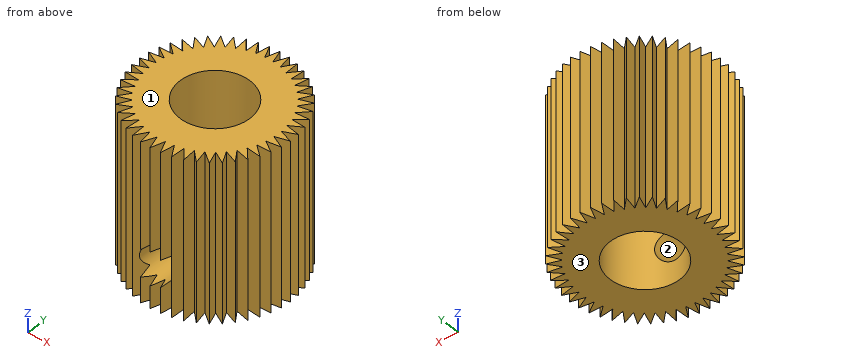
from build123d import *

# Parameters (mm, degrees)
EXTRUDE_1_DEPTH   = 11.4
OTHER_1_OUTLINE_R = 2.5
OTHER_1_DEPTH     = 11.4
SKETCH_9_R        = 1.2


# Read off the part's stored shape, not the designer's step: 孔1
with BuildPart() as part:
    # 草图6 → 凸台-拉伸1 (new body)
    with BuildSketch(Plane.XY):
        Polygon((5.393460046, -0.710062486), (4.490365155, -0.294314082), (5.44, 0), (4.490365155, 0.294314082), (5.393460046, 0.710062486), (4.413533762, 0.877906449), (5.254636495, 1.407975605), (4.261185583, 1.446477594), (5.025904657, 2.081797872), (4.035927337, 1.990299106), (4.711178197, 2.72), (3.741613255, 2.500066049), (4.315842171, 3.311662174), (3.383279134, 2.967056168), (3.84666089, 3.84666089), (2.967056168, 3.383279134), (3.311662174, 4.315842171), (2.500066049, 3.741613255), (2.72, 4.711178197), (1.990299106, 4.035927337), (2.081797872, 5.025904657), (1.446477594, 4.261185583), (1.407975605, 5.254636495), (0.877906449, 4.413533762), (0.710062486, 5.393460046), (0.294314082, 4.490365155), (0, 5.44), (-0.294314082, 4.490365155), (-0.710062486, 5.393460046), (-0.877906449, 4.413533762), (-1.407975605, 5.254636495), (-1.446477594, 4.261185583), (-2.081797872, 5.025904657), (-1.990299106, 4.035927337), (-2.72, 4.711178197), (-2.500066049, 3.741613255), (-3.311662174, 4.315842171), (-2.967056168, 3.383279134), (-3.84666089, 3.84666089), (-3.383279134, 2.967056168), (-4.315842171, 3.311662174), (-3.741613255, 2.500066049), (-4.711178197, 2.72), (-4.035927337, 1.990299106), (-5.025904657, 2.081797872), (-4.261185583, 1.446477594), (-5.254636495, 1.407975605), (-4.413533762, 0.877906449), (-5.393460046, 0.710062486), (-4.490365155, 0.294314082), (-5.44, 0), (-4.490365155, -0.294314082), (-5.393460046, -0.710062486), (-4.413533762, -0.877906449), (-5.254636495, -1.407975605), (-4.261185583, -1.446477594), (-5.025904657, -2.081797872), (-4.035927337, -1.990299106), (-4.711178197, -2.72), (-3.741613255, -2.500066049), (-4.315842171, -3.311662174), (-3.383279134, -2.967056168), (-3.84666089, -3.84666089), (-2.967056168, -3.383279134), (-3.311662174, -4.315842171), (-2.500066049, -3.741613255), (-2.72, -4.711178197), (-1.990299106, -4.035927337), (-2.081797872, -5.025904657), (-1.446477594, -4.261185583), (-1.407975605, -5.254636495), (-0.877906449, -4.413533762), (-0.710062486, -5.393460046), (-0.294314082, -4.490365155), (0, -5.44), (0.294314082, -4.490365155), (0.710062486, -5.393460046), (0.877906449, -4.413533762), (1.407975605, -5.254636495), (1.446477594, -4.261185583), (2.081797872, -5.025904657), (1.990299106, -4.035927337), (2.72, -4.711178197), (2.500066049, -3.741613255), (3.311662174, -4.315842171), (2.967056168, -3.383279134), (3.84666089, -3.84666089), (3.383279134, -2.967056168), (4.315842171, -3.311662174), (3.741613255, -2.500066049), (4.711178197, -2.72), (4.035927337, -1.990299106), (5.025904657, -2.081797872), (4.261185583, -1.446477594), (5.254636495, -1.407975605), (4.413533762, -0.877906449), align=None)
    extrude(amount=EXTRUDE_1_DEPTH)

    # 孔1 outline → 孔1 (cut)
    with BuildSketch(Plane.XY):
        Circle(OTHER_1_OUTLINE_R)
    extrude(amount=OTHER_1_DEPTH, mode=Mode.SUBTRACT)

    # 切除-扫描1: sweep along a path in 草图10
    with BuildLine(Plane(origin=(0, 0, 0), x_dir=(0, 0, -1), z_dir=(1, 0, 0))) as sweep_1_path:
        Line((-2.8, 0), (-2.8, -5.857853696))
    # 草图9 → 切除-扫描1 (sweep, cut)
    with BuildSketch(Plane(origin=(0, 0, 0), x_dir=(1, 0, 0), z_dir=(0, 1, 0))):
        with Locations((0, -2.8)):
            Circle(SKETCH_9_R)
    sweep(path=sweep_1_path.line, mode=Mode.SUBTRACT)


solid = part.part
Read the model definition and answer for the solid it produces. Units are mm, in the model's axes. Face numbers are marked on the shaded views. Coordinates: 2 decimals unless noted, no trailing zeros. Order: outer loops, then holes, each group sorted by start corner. A loop starts at its lowest first (then second) coordinate and runs counter-clockwise, first axis right, second up. Notation, with made-up numbers: (76.5, 62.25) - (130.5, 62.25) arc R11 ccw to (130.5, 80.25) - close; hole circle Ø1 at (15, 57). An arc over 180 degrees is marked (long way). Use one line per item in the form item = value.
(1) For a pull along Z with two mould halves and no side action, classify the marked faces 1, 2 and 3 as pulls with the +Z half, pulls with the -Z half, needs draft (parallel to the pull), parting line crosses it, or undercut.
Computed values:
face_1 = pulls with the +Z half
face_2 = undercut
face_3 = pulls with the -Z half
(2) Section A-A, the plane x = 2.25 is taken. Give the vertices of the cut face in (y, z), then the cut area to 3 significant figures.
Computed values:
outline = (-4.28, 0) - (-1.09, 0) - (-1.09, 11.4) - (-4.28, 11.4) - close; (1.09, 0) - (4.28, 0) - (4.28, 11.4) - (1.09, 11.4) - close
area = 72.7 mm²
(3) Straight lines are drawn through the part: L1, parallel to Z at x = 0, y = -3.95; L2, parallel to Y at x = 3.5, z = 4; L3, parallel to Y at x = 4, z = 8.5. For each, find the intervals that lie inside material, in ascending order.
Computed values:
L1 = 0 to 1.6, 4 to 11.4
L2 = -3.66 to -3.19, -3.01 to 3.01, 3.19 to 3.66
L3 = -3.19 to -2.87, -2.56 to 2.56, 2.87 to 3.19
(4) Given pin 1 Ø1.5 at (x, z) = (-0.5, 3.5) entering from -Y; pin 2 Ø3 at (x, z) = (4, 1.5) entering from +Y; pin 3 Ø4 at (y, z) = (-3, 2.5) entering from -X, each flat-ended and moving along its own axis, determine where each tip first touches the part or whether it passes through.
Computed values:
pin_1 = -5.44
pin_2 = 4.71
pin_3 = -5.25
